Input: part model. Units: mm. Frame: model coordinates. Face numbers are marked on the shaded views. A direction names the side the tool comes from. Give positions to 0.01 mm unless a question says otherwise; leave off trailing zeros. Write each loop counter-clockwise with the first axis right and the second up, starting at its lowest first coordinate (ties: lowest second). Pieces come first, ordered by that corner, then holes. Notation, with made-up numbers: (-19.75, -29) - (20.25, -29) arc R16 ccw to (20.25, -19) - close; hole circle Ø10 at (49, 12.5). An arc over 180 degrees is marked (long way). Use a Markdown table: item, result. Add a question column.
1. Material intervals for probe 1 along Z at (x, y) = (2.1, 0); probe 2 along Z at (x, y) = (2.2, -30) (3 decimals); probe 3 along Y at (x, z) = (1.15, 2.25), sorted ascending.
2. Section query C-C, the plane x = 0.6. Return loops of the section in (y, z) (1 decimal), plus the area to 3 significant figures.
3. Section query A-A, the plane z = 0. Return loops of the section in (x, y) (1 decimal).
4. Set-up query: the marked faces 1 and 2. Return all of +Z, -Z, +X, -X, +Y, -Y with unobstructed straight access to the full face (end or side cutting, diameter ignored); none if empty.
5. Section query B-B, the plane y = 0. Return loops of the section in (x, z) (1 decimal).
6. Section query D-D, the plane y = -20. Return loops of the section in (x, z) (3 decimals).
7. Pin query (flat end, axial travel): pin 1 (1 mm diameter, centred on x = 0.5, y = -1.5, fed in from -Z); pin 2 (1 mm diameter, centred on x = 1.5, y = -24, fed in from -Z). Return the tip coordinate at first contact, or that it passes through.
8. Mould query, pull axis Z, two halves, no side actions, for the marked faces 3, 4 and 5. Classes: released by +Z, released by -Z, zero draft, split by the parting line, or undercut.
Autodesk Inventor part; units mm, degrees
ref_plane "YZ Plane" through (0, 0, 0) normal (1, 0, 0) x (0, 1, 0)
ref_plane "XZ Plane" through (0, 0, 0) normal (0, 1, 0) x (-1, 0, 0)
ref_plane "XY Plane" through (0, 0, 0) normal (0, 0, 1) x (1, 0, 0)
sketch "Sketch2" plane through (0, 0, 0) normal (1, 0, 0) x (0, 1, 0)
  arc A0 (-0.648, -6.3169) -> (-0.648, 6.3169) centre (0, 0) ccw
  line L0 (6.35, 6.35) -> (-34.29, 6.35)
  line L1 (-34.29, 6.35) -> (-34.29, -6.35)
  line L2 (-34.29, -6.35) -> (6.35, -6.35)
  line L3 (6.35, -6.35) -> (6.35, 6.35)
  circle A1 centre (0, 0) radius 1.5875
  line L4 (-34.29, 0) -> (-33.02, 0)
  arc A2 (-31.115, 1.905) -> (-31.115, -1.905) centre (-31.115, 0) ccw
  arc A3 (-31.439, 3.1584) -> (-31.439, -3.1584) centre (-31.115, 0) ccw
  line L5 (-33.02, 0) -> (-13.97, 0)
  arc A4 (-15.875, -1.905) -> (-15.875, 1.905) centre (-15.875, 0) ccw
  line L6 (-15.875, -1.905) -> (-31.115, -1.905)
  line L7 (-15.875, 1.905) -> (-31.115, 1.905)
  line L8 (-0.648, -6.3169) -> (-31.439, -3.1584)
  line L9 (-0.648, 6.3169) -> (-31.439, 3.1584)
  dimension "d16" = 12.7
  dimension "d17" = 40.64
  dimension "d18" = 3.175
  dimension "d19" = 1.27
  dimension "d20" = 3.81
  dimension "d21" = 6.35
  dimension "d22" = 19.05
  dimension "d23" = 3.81
extrude "Extrusion3" add sketch "Sketch2" along normal blind 3.175 contours L8 A3 L9 A0
properties part number "CURM_Caterpillar_leg"
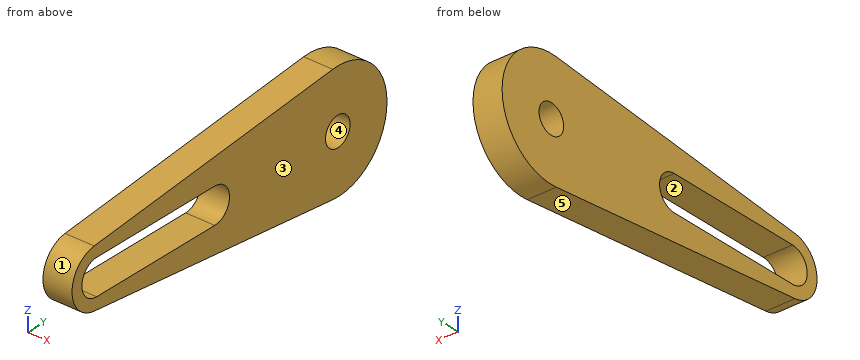
Result sheet:
| question | item | result |
|---|---|---|
| 1 | probe 1 | z = -6.35 to -1.59, 1.59 to 6.35 |
| 1 | probe 2 | z = -3.306 to -1.905, 1.905 to 3.306 |
| 1 | probe 3 | y = -33.36 to 5.94 |
| 2 | outline | (-31.4, -3.2) - (-0.6, -6.3) arc R6.4 ccw (long way) to (-0.6, 6.3) - (-31.4, 3.2) arc R3.2 ccw to start; hole (-31.1, -1.9) - (-15.9, -1.9) arc R1.9 ccw to (-15.9, 1.9) - (-31.1, 1.9) arc R1.9 ccw to start; hole circle Ø3.2 at (0, 0) |
| 2 | area | 300 mm² |
| 3 | outline | (0, -34.3) - (3.2, -34.3) - (3.2, -33) - (0, -33) - close; (0, -14) - (3.2, -14) - (3.2, -1.6) - (0, -1.6) - close; (0, 1.6) - (3.2, 1.6) - (3.2, 6.4) - (0, 6.4) - close |
| 4 | face 1 | +X, -X, -Y |
| 4 | face 2 | +X, -X |
| 5 | outline | (0, -6.4) - (3.2, -6.4) - (3.2, -1.6) - (0, -1.6) - close; (0, 1.6) - (3.2, 1.6) - (3.2, 6.4) - (0, 6.4) - close |
| 6 | outline | (0, -4.332) - (3.175, -4.332) - (3.175, -1.905) - (0, -1.905) - close; (0, 1.905) - (3.175, 1.905) - (3.175, 4.332) - (0, 4.332) - close |
| 7 | pin 1 | stops at z = -6.28 |
| 7 | pin 2 | stops at z = -3.97 |
| 8 | face 3 | zero draft |
| 8 | face 4 | undercut |
| 8 | face 5 | released by -Z |
